```python
from build123d import *

# Parameters (mm, degrees)
SKETCH_1_R          = 4
EXTRUDE_1_DEPTH     = 1
SKETCH_2_R          = 3
EXTRUDE_2_DEPTH     = 6
SKETCH_3_R          = 3
EXTRUDE_3_DEPTH     = 17
SKETCH_4_R          = 7.5
EXTRUDE_4_DEPTH     = 2
SKETCH_5_R          = 5
EXTRUDE_5_DEPTH     = 8
SKETCH_6_R          = 4
EXTRUDE_6_DEPTH     = 54
EXTRUDE_START       = 6
SKETCH_7_R          = 3
EXTRUDE_7_DEPTH     = 6
EXTRUDE_START_2     = 17
SKETCH_8_R          = 3
EXTRUDE_8_DEPTH     = 17
CHAMFER_1_SIZE      = 0.5
CHAMFER_2_SIZE      = 0.5
CUT_EXTRUDE_START   = 2
SKETCH_11_R         = 5
SKETCH_11_R_2       = 4.5
CUT_EXTRUDE_2_DEPTH = 1
SKETCH_12_W         = 4
SKETCH_12_H         = 0.5
CUT_EXTRUDE_3_DEPTH = 5
SKETCH_14_R         = 3
SKETCH_14_R_2       = 1.5
CUT_EXTRUDE_5_DEPTH = 8
SKETCH_15_R         = 3
SKETCH_15_R_2       = 2.5
CUT_EXTRUDE_6_DEPTH = 0.5


with BuildPart() as part:
    # 草图1 → 凸台-拉伸1 (new body)
    with BuildSketch(Plane(origin=(0, 0, 0), x_dir=(0, 0, -1), z_dir=(1, 0, 0))):
        Circle(SKETCH_1_R)
    extrude(amount=EXTRUDE_1_DEPTH)

    # 草图2 → 凸台-拉伸2 (add)
    with BuildSketch(Plane.ZY):
        with Locations(Location((0, 0, 0), (0, 0, 180))):
            Circle(SKETCH_2_R)
    extrude(amount=EXTRUDE_2_DEPTH)

    # 草图3 → 凸台-拉伸3 (add)
    with BuildSketch(Plane.ZY.offset(6)):
        with Locations(Location((0, 0, 0), (0, 0, 180))):
            Circle(SKETCH_3_R)
    extrude(amount=EXTRUDE_3_DEPTH)

    # 草图4 → 凸台-拉伸4 (add)
    with BuildSketch(Plane(origin=(1, 0, 0), x_dir=(0, 0, -1), z_dir=(1, 0, 0))):
        Circle(SKETCH_4_R)
    extrude(amount=EXTRUDE_4_DEPTH)

    # 草图5 → 凸台-拉伸5 (add)
    with BuildSketch(Plane(origin=(3, 0, 0), x_dir=(0, 0, -1), z_dir=(1, 0, 0))):
        Circle(SKETCH_5_R)
    extrude(amount=EXTRUDE_5_DEPTH)

    # 草图6 → 凸台-拉伸6 (add)
    with BuildSketch(Plane(origin=(11, 0, 0), x_dir=(0, 0, -1), z_dir=(1, 0, 0))):
        Circle(SKETCH_6_R)
    extrude(amount=EXTRUDE_6_DEPTH)

    # 草图7 → 凸台-拉伸7 (add)
    with BuildSketch(Plane(origin=(65, 0, 0), x_dir=(0, 0, -1), z_dir=(1, 0, 0)).offset(EXTRUDE_START)):
        Circle(SKETCH_7_R)
    extrude(amount=-EXTRUDE_7_DEPTH)

    # 草图8 → 凸台-拉伸8 (add)
    with BuildSketch(Plane(origin=(71, 0, 0), x_dir=(0, 0, -1), z_dir=(1, 0, 0)).offset(EXTRUDE_START_2)):
        Circle(SKETCH_8_R)
    extrude(amount=-EXTRUDE_8_DEPTH)

    # 倒角1
    chamfer_1_edges = [part.edges().sort_by_distance(p)[0] for p in [
        (65, 0, 4),
    ]]
    chamfer(chamfer_1_edges, length=CHAMFER_1_SIZE)

    # 倒角2
    chamfer_2_edges = [part.edges().sort_by_distance(p)[0] for p in [
        (0, 0, 4),
    ]]
    chamfer(chamfer_2_edges, length=CHAMFER_2_SIZE)

    # 草图11 → 切除-拉伸2 (cut)
    with BuildSketch(Plane(origin=(3, 0, 0), x_dir=(0, 0, -1), z_dir=(1, 0, 0)).offset(CUT_EXTRUDE_START)):
        Circle(SKETCH_11_R)
        Circle(SKETCH_11_R_2, mode=Mode.SUBTRACT)
    extrude(amount=CUT_EXTRUDE_2_DEPTH, mode=Mode.SUBTRACT)

    # 草图12 → 切除-拉伸3 (cut, symmetric)
    with BuildSketch(Plane(origin=(0, 0, 0), x_dir=(1, 0, 0), z_dir=(0, 1, 0))):
        with Locations((47, 3.75)):
            Rectangle(SKETCH_12_W, SKETCH_12_H)
        with Locations((47, -3.75)):
            Rectangle(SKETCH_12_W, SKETCH_12_H)
    extrude(amount=CUT_EXTRUDE_3_DEPTH, both=True, mode=Mode.SUBTRACT)

    # 草图14 → 切除-拉伸5 (cut)
    with BuildSketch(Plane(origin=(88, 0, 0), x_dir=(0, 0, -1), z_dir=(1, 0, 0))):
        Circle(SKETCH_14_R)
        Circle(SKETCH_14_R_2, mode=Mode.SUBTRACT)
    cut_extrude_5 = extrude(amount=-CUT_EXTRUDE_5_DEPTH, mode=Mode.SUBTRACT)

    # 草图15 → 切除-拉伸6 (cut)
    with BuildSketch(Plane(origin=(80, 0, 0), x_dir=(0, 0, -1), z_dir=(1, 0, 0))):
        Circle(SKETCH_15_R)
        Circle(SKETCH_15_R_2, mode=Mode.SUBTRACT)
    cut_extrude_6 = extrude(amount=-CUT_EXTRUDE_6_DEPTH, mode=Mode.SUBTRACT)

    # 镜向2: 切除-拉伸5, 切除-拉伸6 across plane
    add(cut_extrude_5.mirror(Plane(origin=(32.5, 0, 0), x_dir=(0, 0, 1), z_dir=(1, 0, 0))), mode=Mode.SUBTRACT)
    add(cut_extrude_6.mirror(Plane(origin=(32.5, 0, 0), x_dir=(0, 0, 1), z_dir=(1, 0, 0))), mode=Mode.SUBTRACT)


solid = part.part
```
The listing builds one solid part. Answer for the finished solid, in the listing's coordinates (mm). A direction names the side the tool comes from. Round coordinates to 2 decimals unless told otherwise and drop trailing zeros. Order: outer loops, then holes, each group sorted by start corner. A loop starts at its lowest first (then second) coordinate and runs counter-clockwise, first axis right, second up. Notation, with made-up numbers: (-12, 51.25) -> (21, 51.25) arc R27 cw to (21, 89.25) -> close; hole circle Ø1 at (-27, 67.5). An arc over 180 degrees is marked (long way). Answer as CSV lines item,"result".
Q1. A cutting plane is placed at C-C on x = 50. Determine the outline of the cut face in (y, z), plus the area to 3 significant figures.
Computed values:
outline,"circle Ø8 at (0, 0)"
area,"50.3 mm^2"
Q2. Which of the six approach directions +Z, -Z, +X, -X, +Y, -Y give full straight-line access (tool end or side, diameter ignored) to faces 5 (the cylindrical face through (8.46, -4.88, 1.08)), 6 (the flat face through (47, 0, 3.5)), 7 (the cylindrical face through (-7.15, -0.9, -2.86)), 8 (the flat face through (88, 0, 0))?
Computed values:
face 5,"+X"
face 6,"+Z, +Y, -Y"
face 7,"-X"
face 8,"+Z, -Z, +X, +Y, -Y"
Q3. Given pin 1 (1 mm diameter, centred on x = 22, z = -3, fed in from +Y); pin 2 (4 mm diameter, centred on x = 11.5, z = 1, fed in from -Y); pin 3 (3 mm diameter, centred on y = -1, z = 1.5, fed in from -X); pin 4 (4 mm diameter, centred on x = 56.5, z = 1.5, fed in from +Y), each flat-ended and moving along its own axis, determine where each tip first touches the part or whether it passes through.
Computed values:
pin 1,"stops at y = 3.12"
pin 2,"stops at y = -5"
pin 3,"stops at x = -23"
pin 4,"stops at y = 4"
Q4. For a pull along X with two mould halves and no side action, classify faces 1 (the flat face through (1, -3, -3)), 2 (the cylindrical face through (5.49, 4.46, 0.59)), 3 (the cylindrical face through (3.99, -4.88, 1.08)), 4 (the flat face through (47, 0, -3.5)) as +X half, -X half, draft (parallel to the pull), parting line (faces both ways), or undercut.
Computed values:
face 1,"-X half"
face 2,"undercut"
face 3,"draft"
face 4,"undercut"
Q5. A cutting plane is placed at B-B on z = 6. Determine the outline of the cut face in (x, y).
Computed values:
outline,"(1, -4.5) -> (3, -4.5) -> (3, 4.5) -> (1, 4.5) -> close"
Q6. A cutting plane is placed at A-A on x = 9.5. Determine the outline of the cut face in (y, z).
Computed values:
outline,"circle Ø10 at (0, 0)"
Q7. Consider line 1 (X direction, y = 3, z = -4.75); line 2 (X direction, y = -3, z = 1.75); line 3 (Y direction, x = 57, z = 0). Determine where each line is inside the solid, lowest interval first. Write a range as from..to.
Computed values:
line 1,"x = 1..3"
line 2,"x = 0..65"
line 3,"y = -4..4"
